Design review of the part built by this model. Coordinates are the model's own, in mm. Give positions to 0.01 mm unless a question says otherwise; leave off trailing zeros. Order: outer loops, then holes, each group sorted by start corner. A loop starts at its lowest first (then second) coordinate and runs counter-clockwise, first axis right, second up.
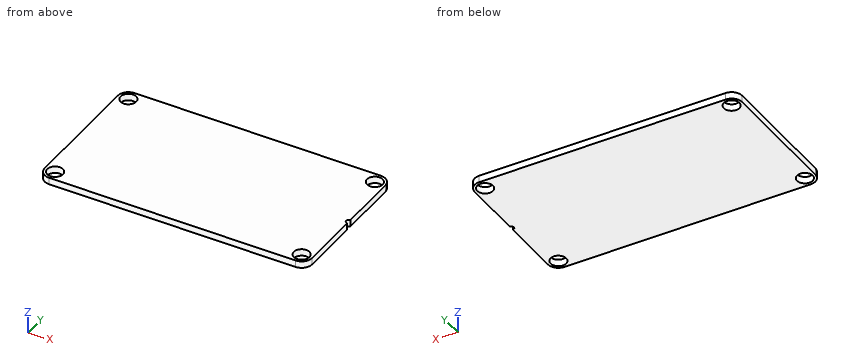
```python
from build123d import *

# Parameters (mm, degrees)
SKETCH_1_W          = 51
SKETCH_1_H          = 28
EXTRUDE_1_DEPTH     = 1.3
SKETCH_2_R          = 1.5
CUT_EXTRUDE_1_DEPTH = 1.3
FILLET_1_R          = 2
FILLET_2_R          = 2
FILLET_3_R          = 2
FILLET_4_R          = 2
SKETCH_4_R          = 0.5
CUT_EXTRUDE_2_DEPTH = 8.8


with BuildPart() as part:
    # Эскиз1 → Бобышка-Вытянуть1 (new body)
    with BuildSketch(Plane.XY):
        Rectangle(SKETCH_1_W, SKETCH_1_H)
    extrude(amount=EXTRUDE_1_DEPTH)

    # Эскиз2 → Вырез-Вытянуть1 (cut)
    with BuildSketch(Plane.XY.offset(1.3)):
        with Locations((23.5, 12)):
            Circle(SKETCH_2_R)
        with Locations((23.5, -12)):
            Circle(SKETCH_2_R)
        with Locations((-23.5, -12)):
            Circle(SKETCH_2_R)
        with Locations((-23.5, 12)):
            Circle(SKETCH_2_R)
    extrude(amount=-CUT_EXTRUDE_1_DEPTH, mode=Mode.SUBTRACT)

    # Скругление1
    fillet_1_edges = [part.edges().sort_by_distance(p)[0] for p in [
        (25.5, 14, 0.65),
    ]]
    fillet(fillet_1_edges, radius=FILLET_1_R)

    # Скругление2
    fillet_2_edges = [part.edges().sort_by_distance(p)[0] for p in [
        (25.5, -14, 0.65),
    ]]
    fillet(fillet_2_edges, radius=FILLET_2_R)

    # Скругление3
    fillet_3_edges = [part.edges().sort_by_distance(p)[0] for p in [
        (-25.5, -14, 0.65),
    ]]
    fillet(fillet_3_edges, radius=FILLET_3_R)

    # Скругление4
    fillet_4_edges = [part.edges().sort_by_distance(p)[0] for p in [
        (-25.5, 14, 0.65),
    ]]
    fillet(fillet_4_edges, radius=FILLET_4_R)

    # Эскиз4 → Вырез-Вытянуть2 (cut)
    with BuildSketch(Plane.XY.offset(1.3)):
        with Locations((25.5, 0)):
            Circle(SKETCH_4_R)
    extrude(amount=-CUT_EXTRUDE_2_DEPTH, mode=Mode.SUBTRACT)


solid = part.part
```
1. For line 1 along Y through (x, z) = (-23.5, 0.8); line 2 along X through (y, z) = (-11.5, 0.35); line 3 along X through (y, z) = (-10.75, 1.1), list the stretches that pass through material, from the lowest coordinate up.
Recorded:
line 1: y = -14 to -13.5, -10.5 to 10.5, 13.5 to 14
line 2: x = -25.5 to -24.91, -22.09 to 22.09, 24.91 to 25.5
line 3: x = -25.5 to -24.33, -22.67 to 22.67, 24.33 to 25.5
2. For pin 1 (2.5 mm diameter, centred on x = -23.5, y = -12, fed in from -Z), flat-tipped, find the tip position at first contact; note if it passes through.
Recorded:
pin 1: passes through
3. Take a section at A-A (z = 1.05). State the section outline as (x, y) points, then the cut area to 3 significant figures.
Recorded:
outline: (-25.5, -12) arc R2 ccw to (-23.5, -14) - (23.5, -14) arc R2 ccw to (25.5, -12) - (25.5, -0.5) arc R0.5 cw to (25.5, 0.5) - (25.5, 12) arc R2 ccw to (23.5, 14) - (-23.5, 14) arc R2 ccw to (-25.5, 12) - close; hole circle Ø3 at (-23.5, -12); hole circle Ø3 at (-23.5, 12); hole circle Ø3 at (23.5, -12); hole circle Ø3 at (23.5, 12)
area: 1,400 mm2
